Source: CAD feature listing. Evaluate the final solid. Frame: model axes, mm. A direction names the side the tool comes from. Round coordinates to 2 decimals unless told otherwise and drop trailing zeros. Loops run counter-clockwise (first coordinate to the right, second up) from the corner with the lowest first, then second, coordinate; pieces in that order, holes last. Notation, with made-up numbers: M 12.25,11.25 L 41.25,11.25 A24 ccw 41.25,28.25 Z; hole C 78.25,78.5 d3. An arc over 180 degrees is marked long. Write each question's results on one line, items separated by ' | '. Start each with the question number.
1. Section A-A on z = 3. Output: boundary loops of the cut face in (x, y), and give its area (3 significant figures).
2. Draft query along X for faces 4 (the cylindrical face through (-25.71, 5.07, -1.24)), 5 (the flat face through (-8, 3, 6.5)), 6 (the flat face through (35, 2, 0)). Return one class per face: released by +X, released by -X, zero draft, split by the parting line, or undercut.
3. Ray query, line 1 (X direction, y = 2.75, z = 0); line 2 (X direction, y = 7.75, z = 0); line 3 (Y direction, x = 6, z = 5.25). Return the intervals inside material, ascending.
4. Section B-B on x = -29.5. Output: boundary loops of the cut face in (y, z), and give its area (3 significant figures).
5. Set-up query: faces 1 (the flat face through (12, 5, 0)), 2 (the flat face through (-32, 5, 0)), 3 (the flat face through (-35, 2, 0)). Return all of +Z, -Z, +X, -X, +Y, -Y with unobstructed straight access to the full face (end or side cutting, diameter ignored); none if empty.
6. Contact query for flat-ended pins moving along their axis: pin 1 Ø3.5 at (x, z) = (-32, 2.5) entering from +Y; pin 2 Ø4 at (y, z) = (8, 1) entering from -X; pin 3 Ø5.5 at (y, z) = (8.5, 3) entering from +X. Output: stop coordinate, or through.
from build123d import *

# Parameters (mm, degrees)
SKETCH1_W           = 70
SKETCH1_H           = 13
BOSS_EXTRUDE1_DEPTH = 5
CUT_EXTRUDE1_DEPTH  = 36.947878936
BOSS_EXTRUDE3_START = 5
SKETCH2_3_W         = 18.390349325
SKETCH2_3_H         = 13
SKETCH2_3_R         = 2
BOSS_EXTRUDE3_DEPTH = 5


with BuildPart() as part:
    # Sketch1 → Boss-Extrude1 (new body)
    with BuildSketch(Plane(origin=(0, 0, 0), x_dir=(1, 0, 0), z_dir=(0, 1, 0))):
        Rectangle(SKETCH1_W, SKETCH1_H)
    extrude(amount=BOSS_EXTRUDE1_DEPTH)

    # Sketch2 → Cut-Extrude1 (cut, through all)
    with BuildSketch(Plane(origin=(0, 5, 0), x_dir=(1, 0, 0), z_dir=(0, 1, 0))):
        with BuildLine():
            ThreePointArc((-22.141309667, 0), (-24.141309667, 2), (-26.141309667, 0))
            Line((-26.141309667, 0), (-22.141309667, 0))
        make_face()
        with BuildLine():
            Line((-22.141309667, 0), (-26.141309667, 0))
            ThreePointArc((-26.141309667, 0), (-24.141309667, -2), (-22.141309667, 0))
        make_face()
        with BuildLine():
            ThreePointArc((-12.141309667, 0), (-14.141309667, 2), (-16.141309667, 0))
            Line((-16.141309667, 0), (-12.141309667, 0))
        make_face()
        with BuildLine():
            Line((-12.141309667, 0), (-16.141309667, 0))
            ThreePointArc((-16.141309667, 0), (-14.141309667, -2), (-12.141309667, 0))
        make_face()
    extrude(amount=-CUT_EXTRUDE1_DEPTH, mode=Mode.SUBTRACT)

    # Sketch2_3 → Boss-Extrude3 (add)
    with BuildSketch(Plane(origin=(0, 5, 0), x_dir=(1, 0, 0), z_dir=(0, 1, 0)).offset(BOSS_EXTRUDE3_START)):
        with Locations((-19.114378827, 0)):
            Rectangle(SKETCH2_3_W, SKETCH2_3_H)
        with Locations(Location((-24.141309667, 0, 0), (0, 0, 270))):
            Circle(SKETCH2_3_R, mode=Mode.SUBTRACT)
        with Locations(Location((-14.141309667, 0, 0), (0, 0, 270))):
            Circle(SKETCH2_3_R, mode=Mode.SUBTRACT)
    extrude(amount=-BOSS_EXTRUDE3_DEPTH)


solid = part.part
Taken from the geometry:
1) outline: M -35,0 L 35,0 L 35,5 L -9.92,5 L -9.92,10 L -28.31,10 L -28.31,5 L -35,5 Z | area: 442 mm^2
2) face 4: undercut | face 5: zero draft | face 6: released by +X
3) line 1: -35 to -26.14, -22.14 to -16.14, -12.14 to 35 | line 2: -28.31 to -26.14, -22.14 to -16.14, -12.14 to -9.92 | line 3: 0 to 5
4) outline: M 0,-6.5 L 5,-6.5 L 5,6.5 L 0,6.5 Z | area: 65.0 mm^2
5) face 1: +Z, -Z, +X, +Y | face 2: +Z, -Z, -X, +Y | face 3: +Z, -Z, -X, +Y, -Y
6) pin 1: y = 5 | pin 2: x = -28.31 | pin 3: x = -9.92
